from build123d import *

# Parameters (mm, degrees)
F0_R     = 28.561798
F0_R_2   = 27.125766
F1_DEPTH = 15
F3_DEPTH = 2.54


with BuildPart() as f1:
    # F0 (on Top) → F1 (new body)
    with BuildSketch(Plane.XY):
        Circle(F0_R)
        Circle(F0_R_2, mode=Mode.SUBTRACT)
    extrude(amount=F1_DEPTH)

    # F2 (on Top) → F3 (join)
    with BuildSketch(Plane.XY):
        with BuildLine():
            ThreePointArc((0, -27.9126), (19.737189, -19.737189), (27.9126, 0))
            ThreePointArc((27.9126, 0), (0, 27.9126), (-27.9126, 0))
            ThreePointArc((-27.9126, 0), (-19.737189, -19.737189), (0, -27.9126))
        make_face()
        with BuildLine():
            ThreePointArc((0, -27.9126), (-19.737189, -19.737189), (-27.9126, 0))
            ThreePointArc((-27.9126, 0), (-31.324946, -31.324946), (0, -27.9126))
        make_face()
    extrude(amount=F3_DEPTH)


solid = f1.part
Design review of the part built by this model. Coordinates are the model's own, in mm. A direction names the side the tool comes from. Coordinates: 2 decimals unless noted, no trailing zeros. Order: outer loops, then holes, each group sorted by start corner. A loop starts at its lowest first (then second) coordinate and runs counter-clockwise, first axis right, second up. Notation, with made-up numbers: (-7, 48) - (18, 48) arc R19 ccw to (18, 84) - close; hole circle Ø2 at (-35, 6). An arc over 180 degrees is marked (long way). Put each result on its own line as item: value.
1) Take a section at B-B, the plane x = 16.5. Give the boundary of the cut face in (y, z), and give its area (3 significant figures).
Response values:
outline: (-23.31, 0) - (23.31, 0) - (23.31, 15) - (21.53, 15) - (21.53, 2.54) - (-21.53, 2.54) - (-21.53, 15) - (-23.31, 15) - close
area: 163 mm²
2) Wall thickness on L1, parallel to X at y = 0, z = 5.75; L2, parallel to X at y = 14, z = 10: over which ranges is each line inside the solid? List them lowest first. Write a range as from..to.
Response values:
L1: x = -28.56..-27.13, 27.13..28.56
L2: x = -24.9..-23.23, 23.23..24.9
3) Take a section at A-A, the plane z = 7.75. Give the boundary of the cut face in (x, y).
Response values:
outline: circle Ø57.12 at (0, 0); hole circle Ø54.25 at (0, 0)
4) Take a section at C-C, the plane y = -15.5. Give the boundary of the cut face in (x, z), and give its area (3 significant figures).
Response values:
outline: (-37.19, 0) - (23.99, 0) - (23.99, 15) - (22.26, 15) - (22.26, 2.54) - (-22.26, 2.54) - (-22.26, 15) - (-23.99, 15) - (-23.99, 2.54) - (-37.19, 2.54) - close
area: 198 mm²
5) The part is to be moulded in two halves that separate along Y. For faces 3 (the face through (0, 0, 2.54)), 4 (the face through (25.3, -10.4, 15)), 5 (the face through (25.873, 8.148, 8.683)), 6 (the face through (15.355, 24.083, 7.395)), say which applies: released by +Y, released by -Y, zero draft, split by the parting line, or undercut.
Response values:
face 3: undercut
face 4: zero draft
face 5: undercut
face 6: split by the parting line
6) Tool access review of faces 1 (the face through (-5, -4, 0)), 2 (the face through (-23, -23, 2.54)): name each direction out of +Z, -Z, +X, -X, +Y, -Y from which nothing blocks a thin tool from reaching the whole face with its end or side.
Response values:
face 1: -Z, +X, -X, +Y, -Y
face 2: +Z, -X, -Y
7) Insertion check: P1, Ø1, axis at y = -20, z = 8, coming from the -X side; P2, Ø4, axis at y = -17, z = 13, coming from the +X side; P3, Ø16.5, axis at x = -1.5, y = -7, coming from the +Z side; P4, Ø1.5, axis at y = -30.5, z = 5.5, coming from the -X side. Each pin has a flat end and moves straight along its axis. Give the tip position at first contact, or say it passes through.
Response values:
P1: stops at x = -20.87
P2: stops at x = 24.31
P3: stops at z = 2.54
P4: passes through
8) Take a section at D-D, the plane x = -24.5. Give the boundary of the cut face in (y, z).
Response values:
outline: (-35.81, 0) - (14.68, 0) - (14.68, 15) - (11.64, 15) - (11.64, 2.54) - (-11.64, 2.54) - (-11.64, 15) - (-14.68, 15) - (-14.68, 2.54) - (-35.81, 2.54) - close
